Verification items for this drawing (mm, ordinates from the low corner). Give positions to 0.01 mm unless a question says otherwise; leave off trailing zeros. Order: outer loops, then holes, each group sorted by start corner. A loop starts at its lowest first (then second) coordinate and runs counter-clockwise, first axis right, second up. Notation, with made-up numbers: M 21,67 L 79,67 A28 cw 79,94 Z; hole C -22.5,54 d9. An arc over 180 degrees is marked long. One line per question, with ' | ' between items. Start each with the question number.
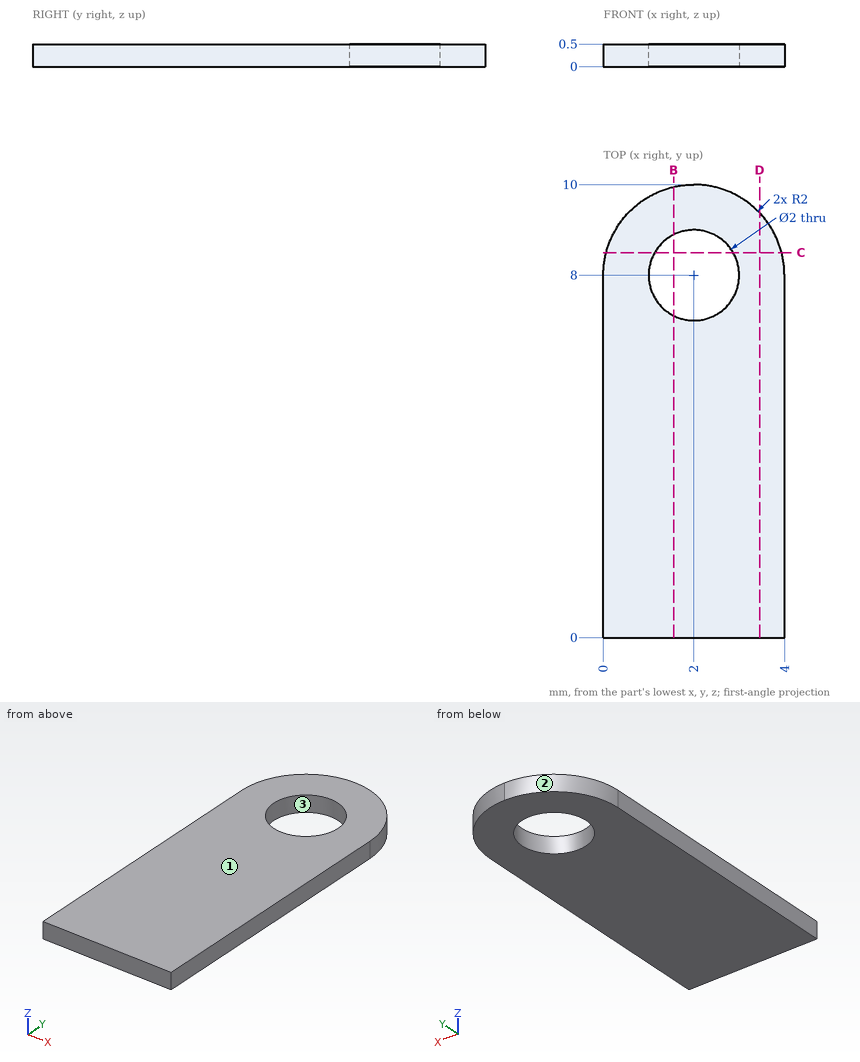
Item 1: Mould release check, pull along Y, two halves, no side actions. Record for the marked faces 1, 2 and 3: released by +Y, released by -Y, zero draft, split by the parting line, or undercut.
Item 2: Cross-section at C-C, the plane y = 8.5. Record the cut outline in (x, z).
Item 3: Cross-section at B-B, the plane x = 1.55. Record the cut outline in (y, z).
Item 4: Cross-section at D-D, the plane x = 3.45. Record the cut outline in (y, z).
Item 5: Material ranges on line 1 along Y through (x, z) = (2, 0.3); line 2 along Y through (x, z) = (1.5, 0.45); line 3 along Y through (x, z) = (0.35, 0.2), recorded low to high.
Outcome:
1) face 1: zero draft | face 2: released by +Y | face 3: undercut
2) outline: M 0.06,0 L 1.13,0 L 1.13,0.5 L 0.06,0.5 Z; M 2.87,0 L 3.94,0 L 3.94,0.5 L 2.87,0.5 Z
3) outline: M 0,0 L 7.11,0 L 7.11,0.5 L 0,0.5 Z; M 8.89,0 L 9.95,0 L 9.95,0.5 L 8.89,0.5 Z
4) outline: M 0,0 L 9.38,0 L 9.38,0.5 L 0,0.5 Z
5) line 1: y = 0 to 7, 9 to 10 | line 2: y = 0 to 7.13, 8.87 to 9.94 | line 3: y = 0 to 9.13
